For this review, take the finished solid that the model builds, in its own axes (mm). A direction names the side the tool comes from. Give positions to 0.01 mm unless a question says otherwise; leave off trailing zeros.
Q1. Mouldability with a two-part tool opening along Y and no side actions: class faces 4 (the flat face through (7, 42, 0)), 5 (the flat face through (0, 0, 6)), 6 (the flat face through (-5.5, 32, 3)) as released by +Y, released by -Y, zero draft, split by the parting line, or undercut.
Q2. For line 1 (Y direction, x = 0.5, z = 1.5); line 2 (X direction, y = 29.5, z = 10); line 3 (X direction, y = 39.5, z = 4.75), list the stretches that pass through material, from the lowest coordinate up.
Q3. Machinability: for faces 1 (the cylindrical face through (-2.718, 5.856, 12.521)), 2 (the flat face through (0, 10, 6)), 3 (the flat face through (-2.3, 10, 14)), which of the approach directions +Z, -Z, +X, -X, +Y, -Y give a long, thin tool a straight path to every point of the face, cutting with its end or side? Answer none if there is none.
Q4. Insertion check: P1, Ø1.5, axis at x = -2.5, y = 46.5, coming from the -Z side; P2, Ø5.5, axis at x = -2, z = 4.5, coming from the +Y side; P3, Ø4.5, axis at y = 30.5, z = 3, coming from the +X side. Each pin has a flat end and moves straight along its axis. Give the tip position at first contact, or say it passes through.
Q5. We need section A-A (z = 2.25). Give the number of separate pieces and of enclosed holes in the cut face, then the cut area to 3 significant figures.
```python
from build123d import *

# Parameters (mm, degrees)
F0_W     = 8.5
F0_H     = 10
F2_ANGLE = 180
F3_DEPTH = 55
F4_DEPTH = 10
F7_DEPTH = 25
F8_DEPTH = 3


with BuildPart() as f2:
    # F0 (on Top) → F2 (revolve)
    with BuildSketch(Plane.XY):
        with BuildLine():
            Line((0, 85), (0, 45))
            Line((0, 45), (5.5, 45))
            Line((5.5, 45), (5.5, 10))
            Line((5.5, 10), (14, 10))
            Line((14, 10), (16, 10))
            add(Edge.make_bspline(
                [(0, 85), (11.4376060665, 85.1000958681), (16.2615635544, 37.3789982498), (16, 10)],
                knots=[0, 0, 0, 0, 76.6876782802, 76.6876782802, 76.6876782802, 76.6876782802], degree=3))
        make_face()
        with Locations((9.75, 5)):
            Rectangle(F0_W, F0_H)
    revolve(axis=Axis((0, 47.5, 0), (0, -1, 0)), revolution_arc=F2_ANGLE)

    # F1 (on Front) → F3 (cut)
    with BuildSketch(Plane.XZ):
        with BuildLine():
            Line((0, 5.5), (0, 0))
            ThreePointArc((0, 0), (3.8890872965, 1.6109127035), (5.5, 5.5))
            Line((5.5, 5.5), (0, 5.5))
        make_face()
        with BuildLine():
            ThreePointArc((5.5, 5.5), (3.8890872965, 1.6109127035), (0, 0))
            Line((0, 0), (5.5, 0))
            Line((5.5, 0), (5.5, 5.5))
        make_face()
        with BuildLine():
            Line((-5.5, 0), (0, 0))
            ThreePointArc((0, 0), (-3.8890872965, 1.6109127035), (-5.5, 5.5))
            Line((-5.5, 5.5), (-5.5, 0))
        make_face()
        with BuildLine():
            ThreePointArc((-5.5, 5.5), (-3.8890872965, 1.6109127035), (0, 0))
            Line((0, 0), (0, 5.5))
            Line((0, 5.5), (-5.5, 5.5))
        make_face()
        with BuildLine():
            Line((-5.5, 5.5), (0, 5.5))
            Line((0, 5.5), (0, 11))
            ThreePointArc((0, 11), (-3.8890872965, 9.3890872965), (-5.5, 5.5))
        make_face()
        with BuildLine():
            Line((0, 11), (0, 5.5))
            Line((0, 5.5), (5.5, 5.5))
            ThreePointArc((5.5, 5.5), (3.8890872965, 9.3890872965), (0, 11))
        make_face()
    extrude(amount=-F3_DEPTH, mode=Mode.SUBTRACT)

    # F1 (on Front) → F4 (join)
    with BuildSketch(Plane.XZ):
        with BuildLine():
            ThreePointArc((5.5, 5.5), (3.8890872965, 1.6109127035), (0, 0))
            Line((0, 0), (5.5, 0))
            Line((5.5, 0), (5.5, 5.5))
        make_face()
        with BuildLine():
            Line((0, 5.5), (0, 0))
            ThreePointArc((0, 0), (3.8890872965, 1.6109127035), (5.5, 5.5))
            Line((5.5, 5.5), (0, 5.5))
        make_face()
        with BuildLine():
            Line((0, 11), (0, 5.5))
            Line((0, 5.5), (5.5, 5.5))
            ThreePointArc((5.5, 5.5), (3.8890872965, 9.3890872965), (0, 11))
        make_face()
        with BuildLine():
            Line((-5.5, 5.5), (0, 5.5))
            Line((0, 5.5), (0, 11))
            ThreePointArc((0, 11), (-3.8890872965, 9.3890872965), (-5.5, 5.5))
        make_face()
        with BuildLine():
            ThreePointArc((-5.5, 5.5), (-3.8890872965, 1.6109127035), (0, 0))
            Line((0, 0), (0, 5.5))
            Line((0, 5.5), (-5.5, 5.5))
        make_face()
        with BuildLine():
            Line((-5.5, 0), (0, 0))
            ThreePointArc((0, 0), (-3.8890872965, 1.6109127035), (-5.5, 5.5))
            Line((-5.5, 5.5), (-5.5, 0))
        make_face()
    extrude(amount=-F4_DEPTH)

    # F6 (on offset) → F7 (cut)
    with BuildSketch(Plane(origin=(0, 0, 14), x_dir=(1, 0, 0), z_dir=(0, 0, -1))):
        with BuildLine():
            Line((0, -3.35), (0, -5))
            Line((0, -5), (0, -6.65))
            ThreePointArc((0, -6.65), (1.166726189, -6.166726189), (1.65, -5))
            ThreePointArc((1.65, -5), (1.166726189, -3.833273811), (0, -3.35))
        make_face()
        with BuildLine():
            ThreePointArc((0, -3.35), (-1.166726189, -3.833273811), (-1.65, -5))
            Line((-1.65, -5), (0, -5))
            Line((0, -5), (0, -3.35))
        make_face()
        with BuildLine():
            Line((0, -5), (-1.65, -5))
            ThreePointArc((-1.65, -5), (-1.166726189, -6.166726189), (0, -6.65))
            Line((0, -6.65), (0, -5))
        make_face()
    extrude(amount=F7_DEPTH, mode=Mode.SUBTRACT)

    # F6 (on offset) → F8 (cut)
    with BuildSketch(Plane(origin=(0, 0, 14), x_dir=(1, 0, 0), z_dir=(0, 0, -1))):
        with BuildLine():
            ThreePointArc((2.85, -5), (0, -2.15), (-2.85, -5))
            ThreePointArc((-2.85, -5), (0, -7.85), (2.85, -5))
        make_face()
        with BuildLine():
            ThreePointArc((0, -6.65), (-1.166726189, -6.166726189), (-1.65, -5))
            ThreePointArc((-1.65, -5), (-1.166726189, -3.833273811), (0, -3.35))
            ThreePointArc((0, -3.35), (1.166726189, -3.833273811), (1.65, -5))
            ThreePointArc((1.65, -5), (1.166726189, -6.166726189), (0, -6.65))
        make_face(mode=Mode.SUBTRACT)
    extrude(amount=F8_DEPTH, mode=Mode.SUBTRACT)


solid = f2.part
```
Computed:
1. face 4: zero draft
1. face 5: released by -Y
1. face 6: undercut
2. line 1: y = 0 to 3.43, 6.57 to 10, 55 to 84.7
2. line 2: x = -11.8 to -3.16, 3.16 to 11.8
2. line 3: x = -13.93 to -5.5, 5.5 to 13.93
3. face 1: +Z
3. face 2: -Z
3. face 3: +Z, -Y
4. P1: stops at z = 9.94
4. P2: stops at y = 84.42
4. P3: stops at x = 15.44
5. separate pieces: 1
5. enclosed holes: 2
5. area: 1,630 mm2
